Model file for the job. Use its own axes, mm. A direction names the side the tool comes from. Give positions to 0.01 mm unless a question says otherwise; leave off trailing zeros. Order: outer loops, then holes, each group sorted by start corner. A loop starts at its lowest first (then second) coordinate and runs counter-clockwise, first axis right, second up. Notation, with made-up numbers: M -17.75,67.5 L 10.25,67.5 A19 cw 10.25,86.5 Z; hole C 10.25,61.25 d2. An arc over 180 degrees is marked long. Return JSON: item names as keys, results as strings. Group by question number.
1. Slice it at C-C on x = -1. List the corners of the cut face in (y, z).
2. Slice it at A-A on z = 10.25. List the corners of the cut face in (x, y), then the cut area to 3 significant figures.
3. 3-axis set-ups, long thin cutter, end or side, ignore diameter. For faces 4 (the face through (-11.27, 7.71, 5.48)), 5 (the face through (-1.09, -13.57, 5.48)), 6 (the face through (12.156, 6, 5)), 7 (the face through (0, 0, 11.112)): which of +Z, -Z, +X, -X, +Y, -Y reach the whole face in a straight line?
4. Wall check: probe 1 along X at (y, z) = (-13, 9.5); probe 2 along X at (y, z) = (17.5, 1.25); probe 3 along X at (y, z) = (12.5, 3). Give the ranges that are in metal, low to high. Write a range as [from, to].
5. Pin check, flat tips, straight feed: pin 1 (1.5 mm diameter, centred on y = -3, z = 4, fed in from +X); pin 2 (4 mm diameter, centred on x = -4, z = 6.5, fed in from +Y); pin 3 (0.7 mm diameter, centred on y = 5.5, z = 5.5, fed in from +X). Stop position of each tip, or through.
6. Slice it at B-B on y = 6. List the corners of the cut face in (x, z), then the cut area to 3 significant figures.
7. Two-plate mould, pull along Y, no slides. Class faces 1 (the face through (19.456, -16.378, 5.478)), 2 (the face through (10.414, 11.774, 5.478)), 3 (the face through (0, 0, 0)): released by +Y, released by -Y, zero draft, split by the parting line, or undercut.
from build123d import *

# Parameters (mm, degrees)
F1_DEPTH = 11.1125


# Not quite as in the source:
# - a length typed as a fraction of an inch, garbled in the dataset ("3 / 203.2 mm" for 3/8 in), is restored


with BuildPart() as f1:
    # F0 (on Top) → F1 (new body)
    with BuildSketch(Plane.XY):
        with BuildLine():
            ThreePointArc((0, 27.0671695471), (-4.5048536548, 25.1556778504), (-8.2258973271, 21.977417171))
            ThreePointArc((-8.2258973271, 21.977417171), (-9.7181261566, 18.698842434), (-9.2097157612, 15.1327075437))
            ThreePointArc((-9.2097157612, 15.1327075437), (-10.6205392688, 11.8246856933), (-10.2093555033, 8.2519613206))
            Line((-10.2093555033, 8.2519613206), (-12.369341217, 7.1464567445))
            Line((-12.369341217, 7.1464567445), (-12.369341217, 4.6386048198))
            Line((-12.369341217, 4.6386048198), (-12.369341217, 4.5682978211))
            ThreePointArc((-12.369341217, 4.5682978211), (-15.5930977879, 3.1185654947), (-17.7027139134, 0.2823972963))
            ThreePointArc((-17.7027139134, 0.2823972963), (-21.0452825194, -1.0603738309), (-23.1384971151, -3.9919692741))
            ThreePointArc((-23.1384971151, -3.9919692741), (-23.9954710425, -8.6613028545), (-23.5336683691, -13.3861117065))
            ThreePointArc((-23.5336683691, -13.3861117065), (-19.6562098094, -16.4130421994), (-15.0192606046, -18.054899429))
            ThreePointArc((-15.0192606046, -18.054899429), (-11.4338171794, -17.7079201351), (-8.5996589687, -15.484556372))
            ThreePointArc((-8.5996589687, -15.484556372), (-5.0294162563, -15.0523544446), (-2.1409380715, -12.9098966718))
            Line((-2.1409380715, -12.9098966718), (0, -14.2561570176))
            Line((0, -14.2561570176), (1.9696742658, -12.9098966718))
            ThreePointArc((1.9696742658, -12.9098966718), (4.9392756736, -15.0084468105), (8.560301624, -15.3410370587))
            ThreePointArc((8.560301624, -15.3410370587), (11.3944598347, -17.5644008218), (14.9799032599, -17.9113801157))
            ThreePointArc((14.9799032599, -17.9113801157), (19.5156578324, -16.3470620723), (23.423301056, -13.563092798))
            ThreePointArc((23.423301056, -13.563092798), (23.8861103651, -8.6849198531), (23.0991397704, -3.8484499608))
            ThreePointArc((23.0991397704, -3.8484499608), (21.0059251747, -0.9168545176), (17.6633565687, 0.4259166096))
            ThreePointArc((17.6633565687, 0.4259166096), (15.4847616458, 3.3168082822), (12.1560195839, 4.739132713))
            Line((12.1560195839, 4.739132713), (12.1560195839, 7.1464567445))
            Line((12.1560195839, 7.1464567445), (9.9960338703, 8.2519613206))
            ThreePointArc((9.9960338703, 8.2519613206), (10.4072176357, 11.8246856933), (8.9963941282, 15.1327075437))
            ThreePointArc((8.9963941282, 15.1327075437), (9.5048045235, 18.698842434), (8.012575694, 21.977417171))
            ThreePointArc((8.012575694, 21.977417171), (4.4155385291, 25.1665589), (0, 27.0671695471))
        make_face()
    extrude(amount=F1_DEPTH)


solid = f1.part
Result:
{
 "1": {"outline": "M -13.63,0 L 26.78,0 L 26.78,11.11 L -13.63,11.11 Z"},
 "2": {"outline": "M -23.53,-13.39 A15.32 ccw -15.02,-18.05 A6.42 ccw -8.6,-15.48 A7.02 ccw -2.14,-12.91 L 0,-14.26 L 1.97,-12.91 A7.02 ccw 8.56,-15.34 A6.42 ccw 14.98,-17.91 A16.78 ccw 23.42,-13.56 A19.2 ccw 23.1,-3.85 A6.42 ccw 17.66,0.43 A7.02 ccw 12.16,4.74 L 12.16,7.15 L 10,8.25 A7.02 ccw 9,15.13 A6.42 ccw 8.01,21.98 A15.14 ccw 0,27.07 A16.08 ccw -8.23,21.98 A6.42 ccw -9.21,15.13 A7.02 ccw -10.21,8.25 L -12.37,7.15 L -12.37,4.57 A7.02 ccw -17.7,0.28 A6.42 ccw -23.14,-3.99 A17.07 ccw Z", "area": "1,300 mm2"},
 "3": {"face 4": "+Z, -Z, -X", "face 5": "+Z, -Z, -Y", "face 6": "+Z, -Z, +X, +Y", "face 7": "+Z, +X, -X, +Y, -Y"},
 "4": {"probe 1": "x = [-23.62, -2.21], [-2, 1.84], [2.05, 23.54]", "probe 2": "x = [-9.78, 9.56]", "probe 3": "x = [-10.49, 10.28]"},
 "5": {"pin 1": "stops at x = 23.06", "pin 2": "stops at y = 26.42", "pin 3": "stops at x = 12.16"},
 "6": {"outline": "M -12.37,0 L 12.16,0 L 12.16,11.11 L -12.37,11.11 Z", "area": "273 mm2"},
 "7": {"face 1": "released by -Y", "face 2": "undercut", "face 3": "zero draft"}
}
